Can you work these out from the drawing? Everything is in mm from the part's minimum corner. A direction names the side the tool comes from. Coordinates: 2 decimals unless noted, no trailing zeros. Order: outer loops, then holes, each group sorted by start corner. A loop starts at its lowest first (then second) coordinate and runs counter-clockwise, first axis right, second up. Notation, with made-up numbers: (-13, 60) - (29, 60) arc R28 ccw to (29, 83) - close; hole circle Ø7 at (54.25, 16.25). An arc over 180 degrees is marked (long way). One line per item, written item: value.
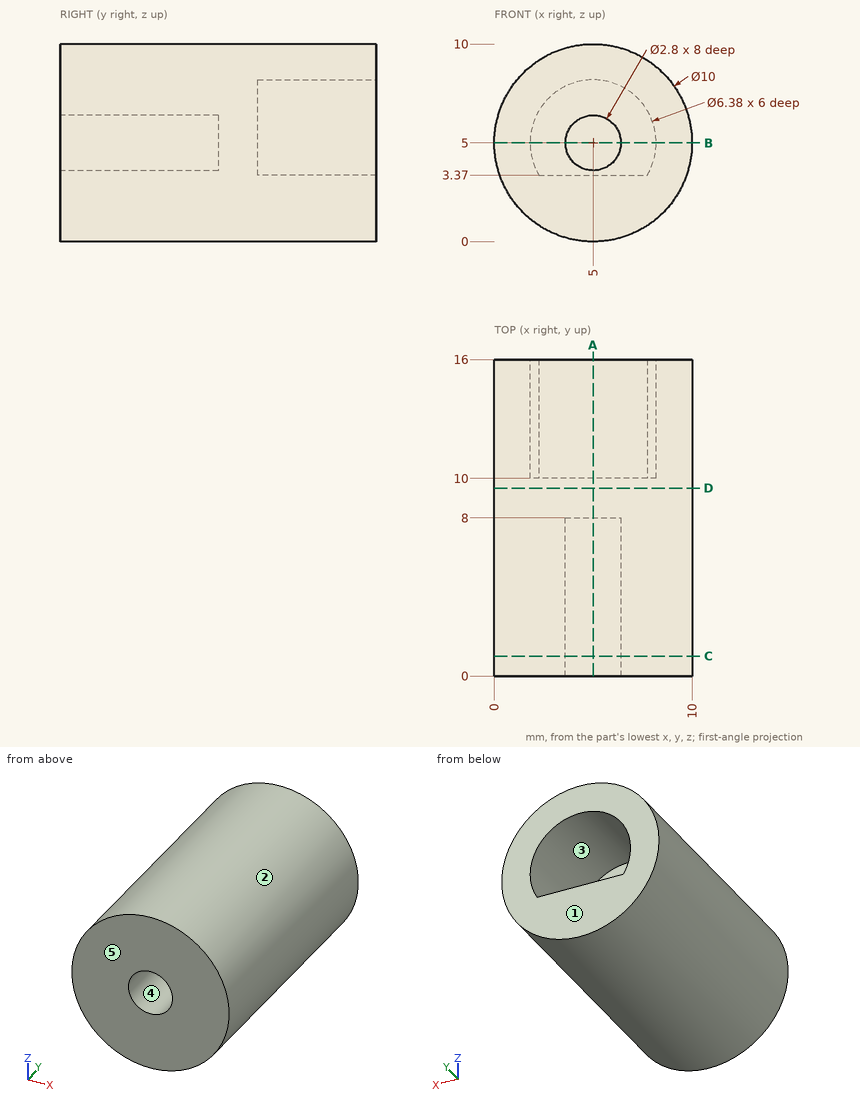
Item 1: I'm going to push flat-ended pins straight in: pin 1 Ø2 at (y, z) = (9.5, 1.5) entering from +X; pin 2 Ø2.5 at (x, z) = (5.5, 6.5) entering from +Y; pin 3 Ø2 at (x, y) = (7.5, 6.5) entering from -Z. Where does each tip first touch, or does it pass through?
Conclusion:
pin 1: x = 9.33
pin 2: y = 10
pin 3: z = 0.23
Item 2: I want a section at C-C on y = 1. Please give me the cut outline in (x, z).
Conclusion:
outline: circle Ø10 at (5, 5); hole circle Ø2.8 at (5, 5)
Item 3: If I drill on probe 1 along Z at (x, y) = (5, 3.5); probe 2 along Z at (x, y) = (5, 14.75); probe 3 along X at (y, z) = (14.75, 5.5), over which ranges is the centre line in solid material (lowest first)?
Conclusion:
probe 1: 0 to 3.6, 6.4 to 10
probe 2: 0 to 3.37, 8.19 to 10
probe 3: 0.03 to 1.85, 8.15 to 9.97
Item 4: I want a section at B-B on z = 5. Please give me the cut outline in (x, y).
Conclusion:
outline: (0, 0) - (3.6, 0) - (3.6, 8) - (6.4, 8) - (6.4, 0) - (10, 0) - (10, 16) - (8.19, 16) - (8.19, 10) - (1.81, 10) - (1.81, 16) - (0, 16) - close
Item 5: I want a section at D-D on y = 9.5. Please give me the cut outline in (x, z).
Conclusion:
outline: circle Ø10 at (5, 5)
Item 6: For the marked faces 4 and 5, which set-ups out of +Z, -Z, +X, -X, +Y, -Y let a thin tool reach every point of the face, with its end or its side?
Conclusion:
face 4: -Y
face 5: +Z, -Z, +X, -X, -Y
Item 7: I want a section at A-A on x = 5. Please give me the cut outline in (y, z), then the cut area to 3 significant figures.
Conclusion:
outline: (0, 0) - (16, 0) - (16, 3.37) - (10, 3.37) - (10, 8.19) - (16, 8.19) - (16, 10) - (0, 10) - (0, 6.4) - (8, 6.4) - (8, 3.6) - (0, 3.6) - close
area: 109 mm²
Item 8: Thinking about a two-plate mould opening in Z: for the marked faces 1, 2 and 3, which applies, pulls with the +Z half, pulls with the -Z half, needs draft (parallel to the pull), parting line crosses it, or undercut?
Conclusion:
face 1: needs draft
face 2: parting line crosses it
face 3: undercut
